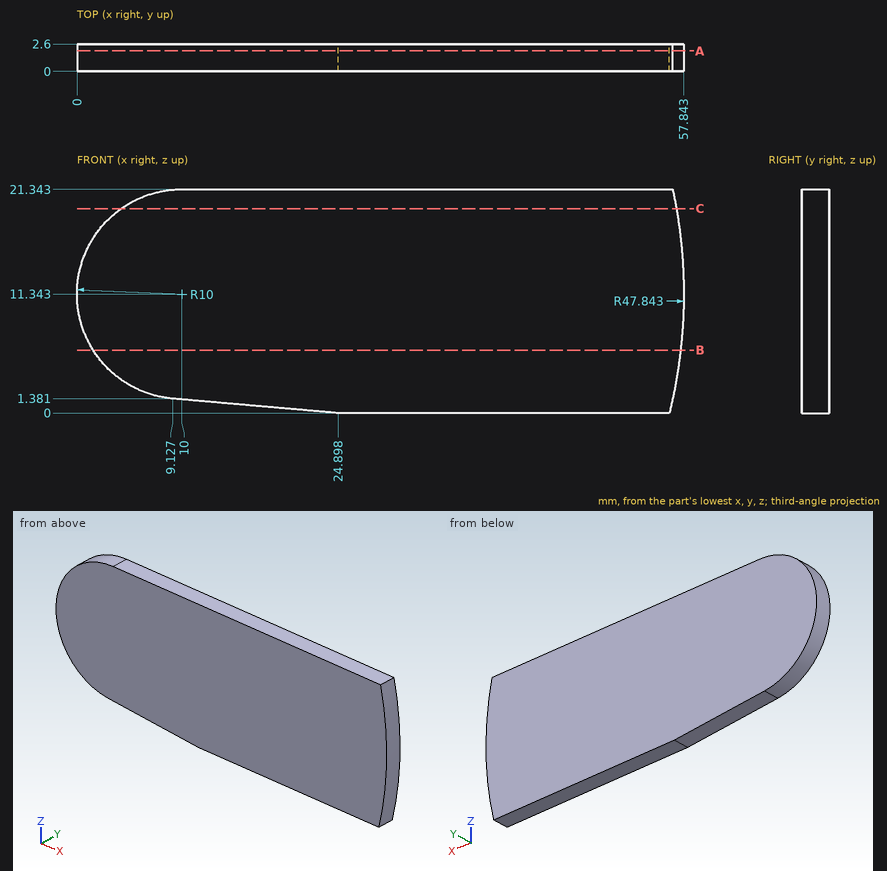
Geometry: see drawing. Coordinates: mm, zero at the bounding-box minimum. Give positions to 0.01 mm unless a question says otherwise; leave off trailing zeros. Loops run counter-clockwise (first coordinate to the right, second up) from the corner with the lowest first, then second, coordinate; pieces in that order, holes last. Notation, with made-up numbers: (-38.75, -18) -> (9.25, -18) arc R19 ccw to (9.25, -2) -> close; hole circle Ø7 at (18.25, 36). An arc over 180 degrees is marked (long way). Use CSV: the item, a comma, the result in double quotes.
(1) Ray query, line 1 along X through (y, z) = (2, 11) (1 decimal); line 2 along X through (y, z) = (2.2, 9.25); line 3 along Z through (x, y) = (4, 0.75) (1 decimal). Return the intervals inside material, ascending. Write a range as [from, to].
From the geometry:
line 1,"[0, 57.8]"
line 2,"[0.22, 57.8]"
line 3,"[3.3, 19.3]"
(2) Cut plane A-A (y = 1.95). Output: boundary loops of the cut face in (x, z) (1 decimal).
From the geometry:
outline,"(9.1, 1.4) -> (24.9, 0) -> (56.5, 0) arc R47.8 ccw to (56.8, 21.3) -> (10, 21.3) arc R10 ccw to start"
(3) Cut plane C-C (z = 19.5). Output: boundary loops of the cut face in (x, y) (1 decimal).
From the geometry:
outline,"(4.2, 0) -> (57.1, 0) -> (57.1, 2.6) -> (4.2, 2.6) -> close"
(4) Cut plane B-B (z = 6). Output: boundary loops of the cut face in (x, y).
From the geometry:
outline,"(1.55, 0) -> (57.54, 0) -> (57.54, 2.6) -> (1.55, 2.6) -> close"
